Input: part model. Units: mm. Frame: model coordinates. Face numbers are marked on the shaded views. A direction names the side the tool comes from. Round coordinates to 2 decimals unless told otherwise and drop trailing zeros. Write each loop counter-clockwise with the first axis right and the second up, starting at its lowest first coordinate (ties: lowest second). Pieces come first, ordered by that corner, then holes. Notation, with made-up numbers: (83.5, -0.75) -> (102.5, -0.75) arc R20 cw to (102.5, 3.25) -> close; hole circle Ø8 at (-4, 13). An arc over 180 degrees is marked (long way). Use CSV: the item, a comma, the result in double quotes.
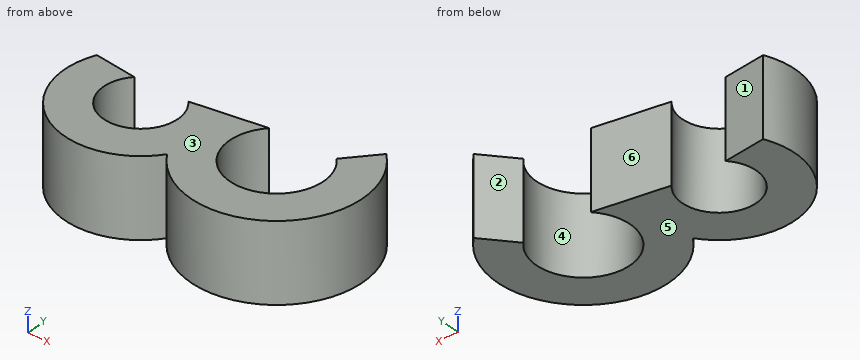
```python
from build123d import *

# Parameters (mm, degrees)
PAD_DEPTH = 4


with BuildPart() as part:
    # Sketch → Pad (new body)
    with BuildSketch(Plane.XY):
        with BuildLine():
            ThreePointArc((-1.4, 2.284523), (0, -0.9), (1.4, 2.284523))
            Line((1.4, 2.284523), (5.126697, 2.842407))
            ThreePointArc((5.126697, 2.842407), (6.876697, -1.2), (8.626697, 2.842407))
            Line((8.626697, 2.842407), (9.926509, 4.371537))
            ThreePointArc((3.204177, -1.223343), (9.691411, -2.181921), (9.926509, 4.371537))
            ThreePointArc((-3.572196, 2.565062), (-1.903119, -2.404136), (3.204177, -1.223343))
            Line((-3.572196, 2.565062), (-1.4, 2.284523))
        make_face()
    extrude(amount=PAD_DEPTH)


solid = part.part
```
Item 1: Section query D-D on z = 2.05. Return the cut outline in (x, y), plus the area to 3 significant figures.
Worked answers:
outline,"(-3.57, 2.57) arc R3.9 ccw to (3.2, -1.22) arc R4.4 ccw (long way) to (9.93, 4.37) -> (8.63, 2.84) arc R2.4 cw (long way) to (5.13, 2.84) -> (1.4, 2.28) arc R1.9 cw (long way) to (-1.4, 2.28) -> close"
area,"50.0 mm²"
Item 2: Section query B-B on y = -1.5. Return the cut outline in (x, z), plus the area to 3 significant figures.
Worked answers:
outline,"(-2.99, 0) -> (2.99, 0) -> (2.99, 4) -> (-2.99, 4) -> close; (3.4, 0) -> (10.35, 0) -> (10.35, 4) -> (3.4, 4) -> close"
area,"51.7 mm²"
Item 3: Pull-direction query (X, two-part tool) for the marked faces 1, 2, 3 and 4; classes: +X half, -X half, draft (parallel to the pull), parting line (faces both ways), or undercut.
Worked answers:
face 1,"undercut"
face 2,"-X half"
face 3,"draft"
face 4,"undercut"
Item 4: Line query: line 1 (X direction, y = 1, z = 2.9); line 2 (X direction, y = -1, z = 1.7); line 3 (X direction, y = 2.25, z = 2.2). Output: solid intervals per line, ascending.
Worked answers:
line 1,"x = -3.9 to -1.9, 1.9 to 4.49, 9.27 to 11.27"
line 2,"x = -3.35 to 5.92, 7.84 to 10.69"
line 3,"x = -3.69 to -1.43, 1.43 to 4.72, 9.03 to 11.15"
Item 5: Section query C-C on x = 0. Return the cut outline in (y, z), plus the area to 3 significant figures.
Worked answers:
outline,"(-2.9, 0) -> (-0.9, 0) -> (-0.9, 4) -> (-2.9, 4) -> close"
area,"8.00 mm²"
Item 6: Section query A-A on y = 1. Return the cut outline in (x, z).
Worked answers:
outline,"(-3.9, 0) -> (-1.9, 0) -> (-1.9, 4) -> (-3.9, 4) -> close; (1.9, 0) -> (4.49, 0) -> (4.49, 4) -> (1.9, 4) -> close; (9.27, 0) -> (11.27, 0) -> (11.27, 4) -> (9.27, 4) -> close"
Item 7: Set-up query: the marked faces 5 and 6. Return all of +Z, -Z, +X, -X, +Y, -Y with unobstructed straight access to the full face (end or side cutting, diameter ignored); none if empty.
Worked answers:
face 5,"-Z, +X, -X, +Y, -Y"
face 6,"+Z, -Z, +Y"
Item 8: First-contact query: pin 1 Ø2 at (y, z) = (-0.5, 2.5) entering from +X; pin 2 Ø1 at (x, z) = (0.5, 1) entering from -Y; pin 3 Ø1 at (y, z) = (-2, 1) entering from +X; pin 4 Ø4.5 at (x, y) = (0, 1) entering from -Z. Flat tips, straight axial feed; report the tip coordinate or a pass-through.
Worked answers:
pin 1,"stops at x = 11.22"
pin 2,"stops at y = -2.9"
pin 3,"stops at x = 10.35"
pin 4,"stops at z = 0"
